Could you check a few things on this model? Use its own coordinates, in mm. A direction names the side the tool comes from. Give positions to 0.01 mm unless a question says otherwise; leave off trailing zeros. Loops run counter-clockwise (first coordinate to the right, second up) from the corner with the lowest first, then second, coordinate; pieces in that order, holes last. Notation, with made-up numbers: M 39,66 L 47,66 A22 cw 47,94 Z; hole C 57,58 d2. An arc over 180 degrees is marked long. Use a Markdown table: item, result. Add a question column.
1) If I drill on line 1 along X through (y, z) = (0, 21.5); line 2 along X through (y, z) = (0, 3.5), over which ranges is the centre line in solid material (lowest first)? Write a range as [from, to].
2) Suppose I cut it at C-C on y = 0. List the corners of the cut face in (x, z) for me, and give its area (4 significant figures).
3) We'd pull the mould along Z, two halves only. Please class faces 4 (the flat face through (-17, 6, 0)), 5 (the cylindrical face through (-2.71, -20.13, 32.797)), 6 (the cylindrical face through (24.4, 24.43, 35.49)), 7 (the flat face through (-17, 6, 70)): +Z half, -Z half, draft (parallel to the pull), parting line (faces both ways), or undercut.
4) Suppose I cut it at D-D on z = 45. List the corners of the cut face in (x, y) for me.
5) Suppose I cut it at B-B on z = 17.5. List the corners of the cut face in (x, y) for me, and give its area (3 significant figures).
6) Suppose I cut it at A-A on x = 0. List the corners of the cut face in (y, z) for me, and give its area (4 significant figures).
7) Which directions (+Z, -Z, +X, -X, +Y, -Y) give clear straight access to the entire face, cutting with the end or side of a thin tool? Please do faces 1 (the flat face through (13, 8, 25)), 2 (the cylindrical face through (-13.887, 10.648, 4.93)), 3 (the cylindrical face through (24.4, -24.43, 35.49)).
8) Will this pin go through, and if not, where does the flat tip stop? pin 1 Ø10.5 at (x, y) = (-5, -7) entering from +Z.
```python
from build123d import *

# Parameters (mm, degrees)
F0_W     = 50
F0_H     = 50
F0_R     = 15
F1_DEPTH = 70
F2_R     = 12.5
F3_DEPTH = 25
F4_R     = 17.5
F5_DEPTH = 45
F6_R     = 17.5
F7_DEPTH = 10
F8_R     = 2


with BuildPart() as f1:
    # F0 (on Top) → F1 (new body)
    with BuildSketch(Plane.XY):
        Rectangle(F0_W, F0_H)
        Circle(F0_R, mode=Mode.SUBTRACT)
    extrude(amount=F1_DEPTH)

    # F2 (on face) → F3 (cut)
    with BuildSketch(Plane.XZ.offset(25)):
        with Locations((0, 45)):
            Circle(F2_R)
    extrude(amount=-F3_DEPTH, mode=Mode.SUBTRACT)

    # F4 (on face) → F5 (cut)
    with BuildSketch(Plane.XY.offset(70)):
        Circle(F4_R)
    extrude(amount=-F5_DEPTH, mode=Mode.SUBTRACT)

    # F6 (on face) → F7 (cut)
    with BuildSketch(Plane(origin=(0, 0, 0), x_dir=(1, 0, 0), z_dir=(0, 0, -1))):
        Circle(F6_R)
    extrude(amount=-F7_DEPTH, mode=Mode.SUBTRACT)

    # F8
    f8_edges = [f1.edges().sort_by_distance(p)[0] for p in [
        (-25, -25, 35),
        (25, -25, 35),
        (25, 25, 35),
        (-25, 25, 35),
    ]]
    fillet(f8_edges, radius=F8_R)


solid = f1.part
```
Answer block:
| question | item | result |
|---|---|---|
| 1 | line 1 | x = [-25, -15], [15, 25] |
| 1 | line 2 | x = [-25, -17.5], [17.5, 25] |
| 2 | outline | M -25,0 L -17.5,0 L -17.5,10 L -15,10 L -15,25 L -17.5,25 L -17.5,70 L -25,70 Z; M 15,10 L 17.5,10 L 17.5,0 L 25,0 L 25,70 L 17.5,70 L 17.5,25 L 15,25 Z |
| 2 | area | 1,125 mm^2 |
| 3 | face 4 | -Z half |
| 3 | face 5 | undercut |
| 3 | face 6 | draft |
| 3 | face 7 | +Z half |
| 4 | outline | M -25,-23 A2 ccw -23,-25 L -12.5,-25 L -12.5,-12.25 A17.5 cw long 12.5,-12.25 L 12.5,-25 L 23,-25 A2 ccw 25,-23 L 25,23 A2 ccw 23,25 L -23,25 A2 ccw -25,23 Z |
| 5 | outline | M -25,-23 A2 ccw -23,-25 L 23,-25 A2 ccw 25,-23 L 25,23 A2 ccw 23,25 L -23,25 A2 ccw -25,23 Z; hole C 0,0 d30 |
| 5 | area | 1,790 mm^2 |
| 6 | outline | M -25,0 L -17.5,0 L -17.5,10 L -15,10 L -15,25 L -17.5,25 L -17.5,32.5 L -25,32.5 Z; M -25,57.5 L -17.5,57.5 L -17.5,70 L -25,70 Z; M 15,10 L 17.5,10 L 17.5,0 L 25,0 L 25,70 L 17.5,70 L 17.5,25 L 15,25 Z |
| 6 | area | 937.5 mm^2 |
| 7 | face 1 | +Z |
| 7 | face 2 | -Z |
| 7 | face 3 | +Z, -Z, +X, -Y |
| 8 | pin 1 | passes through |
